Input: part model. Units: mm. Frame: model coordinates. A direction names the side the tool comes from. Coordinates: 2 decimals unless noted, no trailing zeros. Order: outer loops, then holes, each group sorted by start corner. A loop starts at its lowest first (then second) coordinate and runs counter-clockwise, first axis right, second up. Notation, with made-up numbers: (-2, 62.25) - (3, 62.25) arc R8 cw to (3, 77.25) - close; hole circle Ø2 at (37, 75.25). An arc over 180 degrees is marked (long way). Answer as CSV lines item,"result". Start each with the question number.
Item 1: Section B-B (x = -110). Output: boundary loops of the cut face in (y, z).
Item 2: Material intervals for line 1 along Z through (x, y) = (-111, 41.5); line 2 along Z through (x, y) = (-117, 67); line 3 along X through (y, z) = (44.5, 47.5), sorted ascending.
Item 3: Section C-C (z = 36.5). Output: boundary loops of the cut face in (x, y), and give its area (3 significant figures).
Item 4: Draft query along Z for faces 3 (the flat face through (-108.7, 64.3, 65)), 4 (the flat face through (-105, 41, 153)), 5 (the cylindrical face through (-133.15, 46.5, 32.04)). Return one class per face: +Z half, -Z half, draft (parallel to the pull), parting line (faces both ways), or undercut.
Item 5: Section A-A (y = 57). Output: boundary loops of the cut face in (x, z).
Item 6: Section D-D (y = 49). Output: boundary loops of the cut face in (x, z), and give its area (3 significant figures).
Item 7: First-contact query: pin 1 (6 mm diameter, centred on y = 54.5, z = 115.5, fed in from -X); pin 2 (8 mm diameter, centred on y = 54, z = 18.5, fed in from +X); pin 3 (8 mm diameter, centred on x = -118, y = 53, fed in from +Z); pin 4 (6 mm diameter, centred on y = 37, z = 140, fed in from +X). Flat tips, straight axial feed; report the tip coordinate or a pass-through.
Item 8: Access query for faces 1 (the flat face through (-94, 51, 163)), 2 (the cylindrical face through (-122.66, 46.04, 157.93)). Directions: +Z, -Z, +X, -X, +Y, -Y. A direction counts if a zero-diameter tool reaches every point of the face in a straight line with its end or side. Return the directions, or none.
from build123d import *

# Parameters (mm, degrees)
SKETCH1_R           = 19
BOSS_EXTRUDE1_DEPTH = 65
SKETCH2_R           = 25
BOSS_EXTRUDE2_DEPTH = 3
SKETCH3_R           = 22.5
BOSS_EXTRUDE3_DEPTH = 95
SKETCH4_R           = 20.5
CUT_EXTRUDE1_DEPTH  = 10
SKETCH5_R           = 9.5
SKETCH5_R_2         = 8.5
BOSS_EXTRUDE4_DEPTH = 10


with BuildPart() as part:
    # Sketch1 → Boss-Extrude1 (new body)
    with BuildSketch(Plane.XY):
        with Locations((-114.166758924, 45.66670357)):
            Circle(SKETCH1_R)
    extrude(amount=BOSS_EXTRUDE1_DEPTH)

    # Sketch2 → Boss-Extrude2 (add)
    with BuildSketch(Plane.XY.offset(65)):
        with Locations((-114.166758924, 45.66670357)):
            Circle(SKETCH2_R)
    extrude(amount=BOSS_EXTRUDE2_DEPTH)

    # Sketch3 → Boss-Extrude3 (add)
    with BuildSketch(Plane.XY.offset(68)):
        with Locations((-114.166758924, 45.66670357)):
            Circle(SKETCH3_R)
    extrude(amount=BOSS_EXTRUDE3_DEPTH)

    # Sketch4 → Cut-Extrude1 (cut)
    with BuildSketch(Plane.XY.offset(163)):
        with Locations((-114.166758924, 45.66670357)):
            Circle(SKETCH4_R)
    extrude(amount=-CUT_EXTRUDE1_DEPTH, mode=Mode.SUBTRACT)

    # Sketch5 → Boss-Extrude4 (add)
    with BuildSketch(Plane.XY.offset(153)):
        with Locations((-114.166758924, 45.66670357)):
            Circle(SKETCH5_R)
        with Locations((-114.166758924, 45.66670357)):
            Circle(SKETCH5_R_2, mode=Mode.SUBTRACT)
    extrude(amount=BOSS_EXTRUDE4_DEPTH)


solid = part.part
Determined:
1,outline,"(21.02, 65) - (27.13, 65) - (27.13, 0) - (64.2, 0) - (64.2, 65) - (70.32, 65) - (70.32, 68) - (67.78, 68) - (67.78, 163) - (65.74, 163) - (65.74, 153) - (54.2, 153) - (54.2, 163) - (53.08, 163) - (53.08, 153) - (38.26, 153) - (38.26, 163) - (37.13, 163) - (37.13, 153) - (25.59, 153) - (25.59, 163) - (23.56, 163) - (23.56, 68) - (21.02, 68) - close"
2,line 1,"z = 0 to 153"
2,line 2,"z = 65 to 163"
2,line 3,"x = -133.13 to -95.2"
3,outline,"circle Ø38 at (-114.17, 45.67)"
3,area,"1,130 mm^2"
4,face 3,"-Z half"
4,face 4,"+Z half"
4,face 5,"draft"
5,outline,"(-136.45, 65) - (-129.42, 65) - (-129.42, 0) - (-98.92, 0) - (-98.92, 65) - (-91.88, 65) - (-91.88, 68) - (-94.73, 68) - (-94.73, 163) - (-97.08, 163) - (-97.08, 153) - (-131.25, 153) - (-131.25, 163) - (-133.6, 163) - (-133.6, 68) - (-136.45, 68) - close"
6,outline,"(-138.94, 65) - (-132.87, 65) - (-132.87, 0) - (-95.46, 0) - (-95.46, 65) - (-89.39, 65) - (-89.39, 68) - (-91.92, 68) - (-91.92, 163) - (-93.94, 163) - (-93.94, 153) - (-105.27, 153) - (-105.27, 163) - (-106.35, 163) - (-106.35, 153) - (-121.99, 153) - (-121.99, 163) - (-123.06, 163) - (-123.06, 153) - (-134.39, 153) - (-134.39, 163) - (-136.42, 163) - (-136.42, 68) - (-138.94, 68) - close"
6,area,"6,430 mm^2"
7,pin 1,"stops at x = -135.9"
7,pin 2,"stops at x = -95.67"
7,pin 3,"stops at z = 163"
7,pin 4,"stops at x = -92.39"
8,face 1,"+Z, +X, -X, +Y, -Y"
8,face 2,"+Z"
